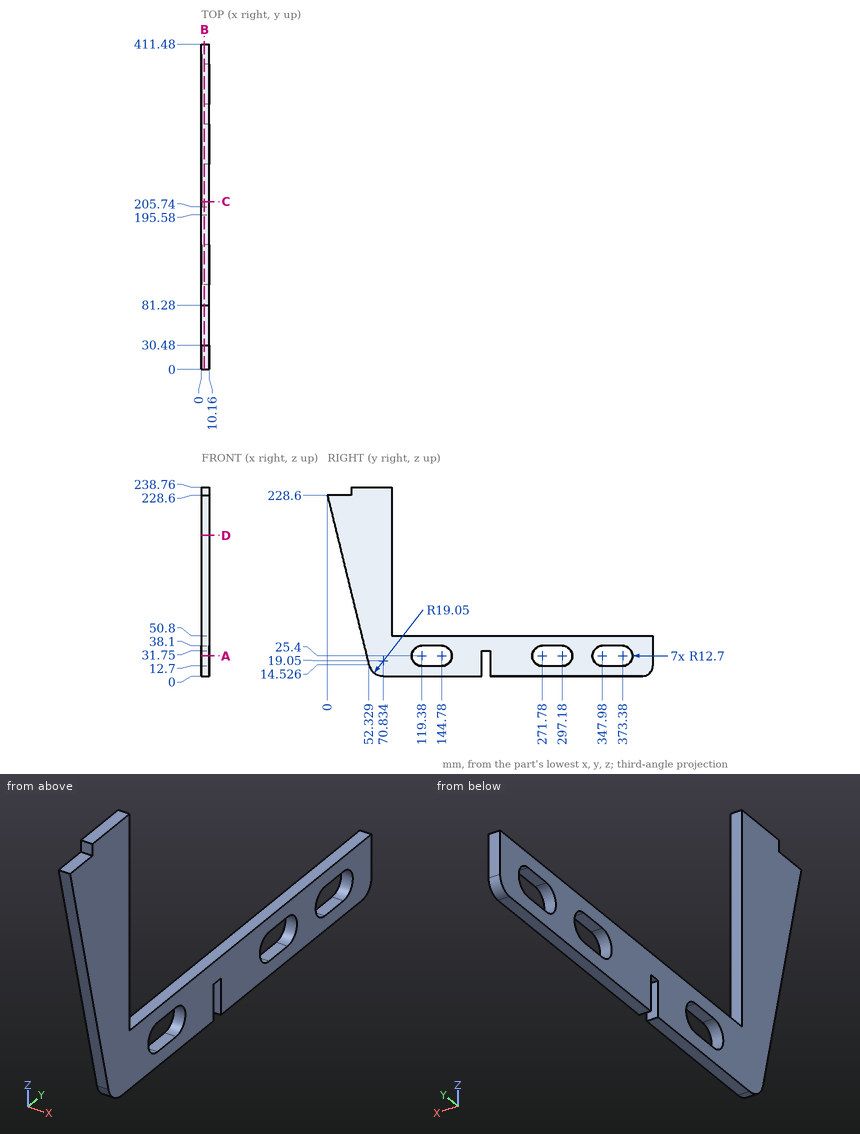
The figure shows three views and two pictorial views of one solid part (mm, origin at its lowest corner). Answer the questions. Give positions to 0.01 mm unless a question says otherwise; leave off trailing zeros. Order: outer loops, then holes, each group sorted by start corner. A loop starts at its lowest first (then second) coordinate and runs counter-clockwise, first axis right, second up. Notation, with made-up numbers: M 65,-39 L 76,-39 A20 ccw 76,-23 Z; hole C 44.25,70 d8. An arc over 180 degrees is marked long. Return JSON: item names as keys, results as strings.
1) Section A-A, the plane z = 25.4 is taken. Write down the section's boundary in (x, y).
Resolved:
{"outline": "M 0,49.67 L 10.16,49.67 L 10.16,106.68 L 0,106.68 Z; M 0,157.48 L 10.16,157.48 L 10.16,195.58 L 0,195.58 Z; M 0,205.74 L 10.16,205.74 L 10.16,259.08 L 0,259.08 Z; M 0,309.88 L 10.16,309.88 L 10.16,335.28 L 0,335.28 Z; M 0,386.08 L 10.16,386.08 L 10.16,411.48 L 0,411.48 Z"}
2) Section B-B, the plane x = 3.75 is taken. Give the number of separate pieces and of enclosed holes in the cut face, plus the area to 3 significant figures.
Resolved:
{"separate pieces": "1", "enclosed holes": "3", "area": "25,600 mm^2"}
3) Each of these flat-tipped pins is pushed along its axis until it touches: pin 1 (1 mm diameter, centred on x = 8, z = 203, fed in from -Y) (1 decimal); pin 2 (3 mm diameter, centred on x = 6.5, y = 128, fed in from +Z); pin 3 (3 mm diameter, centred on x = 4.5, y = 21.5, fed in from +Z). Where does it stop, or does it pass through?
Resolved:
{"pin 1": "y = 6.1", "pin 2": "z = 50.8", "pin 3": "z = 228.6"}
4) Section C-C, the plane y = 212 is taken. Write down the section's boundary in (x, z).
Resolved:
{"outline": "M 0,0 L 10.16,0 L 10.16,50.8 L 0,50.8 Z"}
5) Straight lines are drawn through the part: line 1 along Z through (x, y) = (1.5, 287.5); line 2 along Y through (x, z) = (0.75, 33.5); line 3 along Z through (x, y) = (6.25, 250). For each, find the intervals that lie inside material, in ascending order. Write a range as [from, to].
Resolved:
{"line 1": "[0, 12.7], [38.1, 50.8]", "line 2": "[47.69, 109.6], [154.56, 262], [306.96, 338.2], [383.16, 411.48]", "line 3": "[0, 50.8]"}
6) Section D-D, the plane z = 178 is taken. Write down the section's boundary in (x, y).
Resolved:
{"outline": "M 0,12.37 L 10.16,12.37 L 10.16,81.28 L 0,81.28 Z"}
